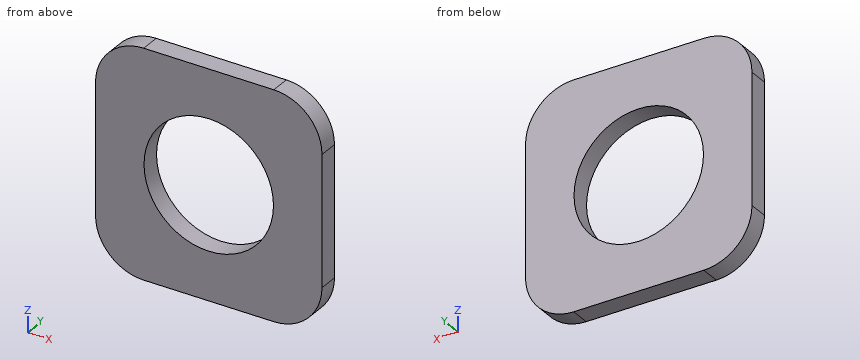
```python
from build123d import *

# Parameters (mm, degrees)
CROQUIS1_W              = 93.98
CROQUIS1_H              = 93.98
SALIENTE_EXTRUIR1_DEPTH = 8.1661
CROQUIS2_R              = 26.8605
CORTAR_EXTRUIR1_DEPTH   = 8.1661
REDONDEO1_R             = 20


with BuildPart() as part:
    # Croquis1 → Saliente-Extruir1 (new body)
    with BuildSketch(Plane(origin=(0, 0, 0), x_dir=(1, 0, 0), z_dir=(0, 1, 0))):
        Rectangle(CROQUIS1_W, CROQUIS1_H)
    extrude(amount=SALIENTE_EXTRUIR1_DEPTH)

    # Croquis2 → Cortar-Extruir1 (cut)
    with BuildSketch(Plane(origin=(0, 8.1661, 0), x_dir=(1, 0, 0), z_dir=(0, 1, 0))):
        Circle(CROQUIS2_R)
    extrude(amount=-CORTAR_EXTRUIR1_DEPTH, mode=Mode.SUBTRACT)

    # Redondeo1
    redondeo1_edges = [part.edges().sort_by_distance(p)[0] for p in [
        (46.99, 4.08305, 46.99),
        (-46.99, 4.08305, 46.99),
        (-46.99, 4.08305, -46.99),
        (46.99, 4.08305, -46.99),
    ]]
    fillet(redondeo1_edges, radius=REDONDEO1_R)


solid = part.part
```
Check sheet for the modelled part. Datum: model origin and axes. Units: mm. Coordinates: 2 decimals unless noted, no trailing zeros. Write each loop counter-clockwise with the first axis right and the second up, starting at its lowest first coordinate (ties: lowest second). Pieces come first, ordered by that corner, then holes. Notation, with made-up numbers: (18.25, 79) -> (55.25, 79) arc R15 ccw to (55.25, 102) -> close; hole circle Ø8 at (85.5, 39). An arc over 180 degrees is marked (long way). Use a Markdown table: item, result.
1. Sectioned sample at B-B (z = 0). Enter the section's corners in (x, y), plus the area to 3 significant figures.
Reported:
| item | result |
|---|---|
| outline | (-46.99, 0) -> (-26.86, 0) -> (-26.86, 8.17) -> (-46.99, 8.17) -> close; (26.86, 0) -> (46.99, 0) -> (46.99, 8.17) -> (26.86, 8.17) -> close |
| area | 329 mm2 |
2. Sectioned sample at C-C (x = -13). Enter the section's corners in (y, z).
Reported:
| item | result |
|---|---|
| outline | (0, -46.99) -> (8.17, -46.99) -> (8.17, -23.51) -> (0, -23.51) -> close; (0, 23.51) -> (8.17, 23.51) -> (8.17, 46.99) -> (0, 46.99) -> close |
3. Sectioned sample at A-A (y = 2.75). Enter the section's corners in (x, z).
Reported:
| item | result |
|---|---|
| outline | (-46.99, -26.99) arc R20 ccw to (-26.99, -46.99) -> (26.99, -46.99) arc R20 ccw to (46.99, -26.99) -> (46.99, 26.99) arc R20 ccw to (26.99, 46.99) -> (-26.99, 46.99) arc R20 ccw to (-46.99, 26.99) -> close; hole circle Ø53.72 at (0, 0) |
4. Scan lines: line 1 along X through (y, z) = (5.5, 0); line 2 along Z through (x, y) = (-17.5, 6.5). Record each from-to range of solid material in increasing order.
Reported:
| item | result |
|---|---|
| line 1 | x = -46.99 to -26.86, 26.86 to 46.99 |
| line 2 | z = -46.99 to -20.38, 20.38 to 46.99 |
5. Sectioned sample at D-D (z = -39). Enter the section's corners in (x, y), plus the area to 3 significant figures.
Reported:
| item | result |
|---|---|
| outline | (-42.98, 0) -> (42.98, 0) -> (42.98, 8.17) -> (-42.98, 8.17) -> close |
| area | 702 mm2 |
